```python
from build123d import *

# Parameters (mm, degrees)
SKETCH_R      = 2.5
PAD_DEPTH     = 5
SKETCH001_R   = 6.5
SKETCH001_R_2 = 2.5
PAD001_DEPTH  = 1
SKETCH002_R   = 2.5
PAD002_DEPTH  = 4


with BuildPart() as part:
    # Sketch → Pad (new body)
    with BuildSketch(Plane.XY):
        with BuildLine():
            Line((6, 2.397916), (6, -2.397916))
            ThreePointArc((6, 2.397916), (-5.5, 0), (6, -2.397916))
        make_face()
        Circle(SKETCH_R, mode=Mode.SUBTRACT)
    extrude(amount=-PAD_DEPTH)

    # Sketch001 (on Face5 of Pad) → Pad001 (join)
    with BuildSketch(Plane(origin=(0, 0, -5), x_dir=(1, 0, 0), z_dir=(0, 0, -1))):
        Circle(SKETCH001_R)
        Circle(SKETCH001_R_2, mode=Mode.SUBTRACT)
    extrude(amount=PAD001_DEPTH)

    # Sketch002 (on Face8 of Pad001) → Pad002 (join)
    with BuildSketch(Plane(origin=(0, 0, -6), x_dir=(1, 0, 0), z_dir=(0, 0, -1))):
        with BuildLine():
            ThreePointArc((-6, -2.397916), (5.5, 0), (-6, 2.397916))
            Line((-6, 2.397916), (-6, -2.397916))
        make_face()
        Circle(SKETCH002_R, mode=Mode.SUBTRACT)
    extrude(amount=PAD002_DEPTH)


solid = part.part
```
Check sheet for the modelled part. Datum: model origin and axes. Units: mm. A direction names the side the tool comes from. Round coordinates to 2 decimals unless told otherwise and drop trailing zeros. Order: outer loops, then holes, each group sorted by start corner. A loop starts at its lowest first (then second) coordinate and runs counter-clockwise, first axis right, second up. Notation, with made-up numbers: (-14.5, 22) - (18.5, 22) arc R32 cw to (18.5, 49) - close; hole circle Ø7 at (72.5, 1). An arc over 180 degrees is marked (long way). Answer as CSV lines item,"result". Start each with the question number.
1) Tool access check on faces 1 (the face through (6, 0, -2)), 2 (the face through (6, 0, -6)), 3 (the face through (-6, 0, -5)), 4 (the face through (3, 0, 0)), 5 (the face through (-6, 0, -8)). Record the directions out of +Z, -Z, +X, -X, +Y, -Y that give a thin tool (end or side, any length) a straight path to the whole face; none if there is none.
2) Scan lines: probe 1 along Y at (x, z) = (0, -5.7); probe 2 along X at (y, z) = (0, -8.6). Record each from-to range of solid material in increasing order.
3) Depth check by flat-ended pin: pin 1 (4 mm diameter, centred on x = -4, z = -5.5, fed in from +Y); pin 2 (4 mm diameter, centred on x = 0, y = 0, fed in from -Z); pin 3 (2 mm diameter, centred on y = 0.5, z = -7.5, fed in from -X); pin 4 (4 mm diameter, centred on y = -4.5, z = -3.5, fed in from +X). Enter the tip coordinate at first touch or a pass-through.
4) Section check C-C (z = -8). Record the cut outline in (x, y).
5) Section check D-D (y = 5.75). Record the cut outline in (x, z), then the cut area to 3 significant figures.
6) Section check B-B (x = 0.5). Record the cut outline in (y, z), then the cut area to 3 significant figures.
7) Section check A-A (y = 0). Record the cut outline in (x, z).
Determined:
1,face 1,"+Z, +X, +Y, -Y"
1,face 2,"-Z"
1,face 3,"+Z"
1,face 4,"+Z, +X, -X, +Y, -Y"
1,face 5,"-Z, -X, +Y, -Y"
2,probe 1,"-6.5 to -2.5, 2.5 to 6.5"
2,probe 2,"-6 to -2.5, 2.5 to 5.5"
3,pin 1,"y = 6.18"
3,pin 2,"through"
3,pin 3,"x = -6"
3,pin 4,"x = 5.95"
4,outline,"(-6, -2.4) arc R6 ccw (long way) to (-6, 2.4) - close; hole circle Ø5 at (0, 0)"
5,outline,"(-3.03, -6) - (-2.21, -6) - (-2.21, -10) - (1.21, -10) - (1.21, -6) - (3.03, -6) - (3.03, -5) - (2.21, -5) - (2.21, 0) - (-1.21, 0) - (-1.21, -5) - (-3.03, -5) - close"
5,area,"36.9 mm^2"
6,outline,"(-6.48, -6) - (-5.92, -6) - (-5.92, -10) - (-2.45, -10) - (-2.45, 0) - (-6, 0) - (-6, -5) - (-6.48, -5) - close; (2.45, -10) - (5.92, -10) - (5.92, -6) - (6.48, -6) - (6.48, -5) - (6, -5) - (6, 0) - (2.45, 0) - close"
6,area,"71.3 mm^2"
7,outline,"(-6.5, -6) - (-6, -6) - (-6, -10) - (-2.5, -10) - (-2.5, 0) - (-5.5, 0) - (-5.5, -5) - (-6.5, -5) - close; (2.5, -10) - (5.5, -10) - (5.5, -6) - (6.5, -6) - (6.5, -5) - (6, -5) - (6, 0) - (2.5, 0) - close"
